```python
from build123d import *

# Parameters (mm, degrees)
F0_W     = 45.72
F0_H     = 56.769
F0_R     = 2.5
F0_R_2   = 1.143
F0_W_2   = 24.13
F0_H_2   = 25.4
F1_DEPTH = 3.81


with BuildPart() as f1:
    # F0 (on Top) → F1 (new body)
    with BuildSketch(Plane.XY):
        Polygon((5.469258, 41.86581), (-17.390742, 41.86581), (-23.740742, 41.86581), (-23.740742, -47.508215), (-23.740742, -72.908215), (39.759258, -72.908215), (39.759258, 41.86581), (33.409258, 41.86581), (10.549258, 41.86581), (12.454258, 38.566253), (3.564258, 38.566253), align=None)
        with Locations((8.009258, -36.071789)):
            Rectangle(F0_W, F0_H, mode=Mode.SUBTRACT)
        with Locations((1.659258, 3.76581)):
            Circle(F0_R, mode=Mode.SUBTRACT)
        with Locations((-6.976742, 22.889307)):
            Circle(F0_R_2, mode=Mode.SUBTRACT)
        with Locations((8.009258, 22.889307)):
            Rectangle(F0_W_2, F0_H_2, mode=Mode.SUBTRACT)
        with Locations((14.359258, 3.76581)):
            Circle(F0_R, mode=Mode.SUBTRACT)
        with Locations((22.995258, 22.889307)):
            Circle(F0_R_2, mode=Mode.SUBTRACT)
    extrude(amount=F1_DEPTH)


solid = f1.part
```
Geometry check sheet. Reference: the model listing, model coordinates, mm. A direction names the side the tool comes from. Coordinates: 2 decimals unless noted, no trailing zeros. Order: outer loops, then holes, each group sorted by start corner. A loop starts at its lowest first (then second) coordinate and runs counter-clockwise, first axis right, second up. Notation, with made-up numbers: M -39,79.25 L 11,79.25 A24 cw 11,93.25 Z; hole C 10.25,-28.75 d7. An arc over 180 degrees is marked long. Answer as a JSON object with one key per item and string values.
Q1. Tool access check on faces 1 (the flat face through (25, 41.866, 2)), 2 (the flat face through (8, 35.589, 2)). Record the directions out of +Z, -Z, +X, -X, +Y, -Y that give a thin tool (end or side, any length) a straight path to the whole face; none if there is none.
Results are:
{"face 1": "+Z, -Z, +X, -X, +Y", "face 2": "+Z, -Z"}
Q2. Cross-section at D-D on x = 15. Record the cut outline in (y, z).
Results are:
{"outline": "M -72.91,0 L -64.46,0 L -64.46,3.81 L -72.91,3.81 Z; M -7.69,0 L 1.35,0 L 1.35,3.81 L -7.69,3.81 Z; M 6.18,0 L 10.19,0 L 10.19,3.81 L 6.18,3.81 Z; M 35.59,0 L 41.87,0 L 41.87,3.81 L 35.59,3.81 Z"}
Q3. Cross-section at C-C on z = 1.55. Record the cut outline in (x, y), and give its area (3 significant figures).
Results are:
{"outline": "M -23.74,-72.91 L 39.76,-72.91 L 39.76,41.87 L 10.55,41.87 L 12.45,38.57 L 3.56,38.57 L 5.47,41.87 L -23.74,41.87 Z; hole M -14.85,-64.46 L 30.87,-64.46 L 30.87,-7.69 L -14.85,-7.69 Z; hole C -6.98,22.89 d2.29; hole M -4.06,10.19 L 20.07,10.19 L 20.07,35.59 L -4.06,35.59 Z; hole C 1.66,3.77 d5; hole C 14.36,3.77 d5; hole C 23,22.89 d2.29", "area": "4,010 mm²"}
Q4. Cross-section at B-B on y = -16.5. Record the cut outline in (x, z).
Results are:
{"outline": "M -23.74,0 L -14.85,0 L -14.85,3.81 L -23.74,3.81 Z; M 30.87,0 L 39.76,0 L 39.76,3.81 L 30.87,3.81 Z"}
Q5. Release check for a two-part mould opening along X. For faces 3 (the flat face through (8, -64.456, 2)), 4 (the cylindrical face through (2.813, 1.548, 1.878)), 5 (the flat face through (8, -72.908, 2)), 6 (the flat face through (39.759, -16, 2)) record: released by +X, released by -X, zero draft, split by the parting line, or undercut.
Results are:
{"face 3": "undercut", "face 4": "undercut", "face 5": "zero draft", "face 6": "released by +X"}
Q6. Cross-section at A-A on y = 13.5. Record the cut outline in (x, z), and give its area (3 significant figures).
Results are:
{"outline": "M -23.74,0 L -4.06,0 L -4.06,3.81 L -23.74,3.81 Z; M 20.07,0 L 39.76,0 L 39.76,3.81 L 20.07,3.81 Z", "area": "150 mm²"}
Q7. Depth check by flat-ended pin: pin 1 Ø1.5 at (x, y) = (28, 15) entering from -Z; pin 2 Ø2 at (x, z) = (7.5, 2.5) entering from +Y; pin 3 Ø1.8 at (x, y) = (-6.98, 22.89) entering from -Z. Enter the tip coordinate at first touch or a pass-through.
Results are:
{"pin 1": "stops at z = 0", "pin 2": "stops at y = 38.57", "pin 3": "passes through"}
Q8. Scan lines: line 1 (X direction, y = 4, z = 1.2); line 2 (Y direction, x = -7, z = 1.65); line 3 (X direction, y = -54, z = 0.7). Record each from-to range of solid material in increasing order.
Results are:
{"line 1": "x = -23.74 to -0.83, 4.15 to 11.87, 16.85 to 39.76", "line 2": "y = -72.91 to -64.46, -7.69 to 21.75, 24.03 to 41.87", "line 3": "x = -23.74 to -14.85, 30.87 to 39.76"}
